```python
from build123d import *

# Parameters (mm, degrees)
F0_W     = 63.5
F0_H     = 63.5
F1_DEPTH = 63.5
F2_W     = 31.75
F2_H     = 12.7
F3_DEPTH = 63.5
F4_W     = 19.05
F4_H     = 19.05
F5_DEPTH = 63.5
F7_DEPTH = 63.5


with BuildPart() as f1:
    # F0 (on Top) → F1 (new body)
    with BuildSketch(Plane.XY):
        with Locations((-28.497959, -34.744633)):
            Rectangle(F0_W, F0_H)
    extrude(amount=F1_DEPTH)

    # F2 (on face) → F3 (cut)
    with BuildSketch(Plane.XY.offset(63.5)):
        with Locations((-44.372959, -47.444633)):
            Rectangle(F2_W, F2_H)
        with Locations((-44.372959, -22.044633)):
            Rectangle(F2_W, F2_H)
    extrude(amount=-F3_DEPTH, mode=Mode.SUBTRACT)

    # F4 (on face) → F5 (cut)
    with BuildSketch(Plane.YZ.offset(3.252041)):
        Polygon((-28.394633, 31.75), (-34.744633, 31.75), (-34.744633, 0), (-2.994633, 0), (-2.994633, 31.75), align=None)
        with Locations((-18.869633, 47.625)):
            Rectangle(F4_W, F4_H)
    extrude(amount=-F5_DEPTH, mode=Mode.SUBTRACT)

    # F6 (on face) → F7 (cut)
    with BuildSketch(Plane.XZ.offset(66.494633)):
        Polygon((-47.547959, 50.8), (-47.547959, 12.7), (-9.447959, 17.444041), (-9.447959, 44.424161), align=None)
    extrude(amount=-F7_DEPTH, mode=Mode.SUBTRACT)


solid = f1.part
```
Source: CAD feature listing. Evaluate the final solid. Frame: model axes, mm. A direction names the side the tool comes from. Coordinates: 2 decimals unless noted, no trailing zeros. Write each loop counter-clockwise with the first axis right and the second up, starting at its lowest first coordinate (ties: lowest second). Pieces come first, ordered by that corner, then holes. Notation, with made-up numbers: (19.25, 59) - (57.25, 59) arc R17 ccw to (57.25, 71) - close; hole circle Ø1 at (31, 57). An arc over 180 degrees is marked (long way). Answer as a JSON object with one key per item and string values.
Q1. Section query B-B, the plane y = -56.5. Output: boundary loops of the cut face in (x, z), plus the area to 3 significant figures.
Ans:
{"outline": "(-60.25, 0) - (3.25, 0) - (3.25, 63.5) - (-60.25, 63.5) - close; hole (-47.55, 12.7) - (-9.45, 17.44) - (-9.45, 44.42) - (-47.55, 50.8) - close", "area": "2,790 mm2"}
Q2. First-contact query: pin 1 Ø16 at (x, z) = (-39.5, 16.5) entering from +Y; pin 2 Ø10 at (x, y) = (-2.5, -14) entering from -Z; pin 3 Ø1.5 at (x, z) = (-11.5, 33) entering from +Y; pin 4 Ø5 at (y, z) = (-23, 61) entering from -X. Flat tips, straight axial feed; report the tip coordinate or a pass-through.
Ans:
{"pin 1": "stops at y = -34.74", "pin 2": "stops at z = 31.75", "pin 3": "passes through", "pin 4": "stops at x = -28.5"}
Q3. Section query A-A, the plane z = 42. Output: boundary loops of the cut face in (x, y), plus the area to 3 significant figures.
Ans:
{"outline": "(-60.25, -66.49) - (-47.55, -66.49) - (-47.55, -53.79) - (-60.25, -53.79) - close; (-60.25, -41.09) - (-47.55, -41.09) - (-47.55, -28.39) - (-60.25, -28.39) - close; (-60.25, -9.34) - (-47.55, -9.34) - (-47.55, -2.99) - (-60.25, -2.99) - close; (-9.45, -66.49) - (3.25, -66.49) - (3.25, -28.39) - (-9.45, -28.39) - close; (-9.45, -9.34) - (3.25, -9.34) - (3.25, -2.99) - (-9.45, -2.99) - close", "area": "968 mm2"}
Q4. Section query C-C, the plane x = -20. Output: boundary loops of the cut face in (y, z).
Ans:
{"outline": "(-66.49, 0) - (-34.74, 0) - (-34.74, 16.13) - (-66.49, 16.13) - close; (-66.49, 46.19) - (-28.39, 46.19) - (-28.39, 57.15) - (-9.34, 57.15) - (-9.34, 46.19) - (-2.99, 46.19) - (-2.99, 63.5) - (-66.49, 63.5) - close"}
Q5. Material intervals for line 1 (Y direction, x = -53.5, z = 48); line 2 (Y direction, x = -29, z = 13); line 3 (X direction, y = -35.5, z = 36), sorted ascending. Write a range as [from, to].
Ans:
{"line 1": "y = [-66.49, -53.79], [-41.09, -28.39], [-9.34, -2.99]", "line 2": "y = [-66.49, -53.79], [-41.09, -34.74]", "line 3": "x = [-60.25, -47.55], [-9.45, 3.25]"}
Q6. Section query D-D, the plane z = 34. Output: boundary loops of the cut face in (x, y).
Ans:
{"outline": "(-60.25, -66.49) - (-47.55, -66.49) - (-47.55, -53.79) - (-60.25, -53.79) - close; (-60.25, -41.09) - (-47.55, -41.09) - (-47.55, -28.39) - (-60.25, -28.39) - close; (-60.25, -15.69) - (-47.55, -15.69) - (-47.55, -2.99) - (-60.25, -2.99) - close; (-9.45, -66.49) - (3.25, -66.49) - (3.25, -2.99) - (-9.45, -2.99) - close"}
Q7. Draft query along Z for faces 1 (the flat face through (-54, -9, 31.75)), 2 (the flat face through (-22, -34, 63.5)), 3 (the flat face through (-60.248, -60, 31)), 4 (the flat face through (-28.231, -47.711, 47.567)). Return one class per face: released by +Z, released by -Z, zero draft, split by the parting line, or undercut.
Ans:
{"face 1": "released by -Z", "face 2": "released by +Z", "face 3": "zero draft", "face 4": "undercut"}
Q8. Set-up query: faces 5 (the flat face through (-47.548, -60, 32)), 6 (the flat face through (-3, -19, 38.1)), 7 (the flat face through (-28, -34.745, 13)), 8 (the flat face through (-48, -41.095, 32)). Return all of +Z, -Z, +X, -X, +Y, -Y with unobstructed straight access to the full face (end or side cutting, diameter ignored); none if empty.
Ans:
{"face 5": "+Y, -Y", "face 6": "+X, -X", "face 7": "-Z, +X, -X, +Y", "face 8": "+Z, -Z, -X"}
